Check sheet for the modelled part. Datum: model origin and axes. Units: mm. A direction names the side the tool comes from. Round coordinates to 2 decimals unless told otherwise and drop trailing zeros. Write each loop counter-clockwise with the first axis right and the second up, starting at its lowest first coordinate (ties: lowest second). Pieces come first, ordered by that corner, then holes.
Item 1: Section check C-C, the plane x = 0. Record the cut outline in (y, z).
Item 2: Section check A-A, the plane x = -9.5. Record the cut outline in (y, z).
Item 3: Section check D-D, the plane y = -1. Record the cut outline in (x, z).
Item 4: Depth check by flat-ended pin: pin 1 (0.6 mm diameter, centred on x = -14.5, z = 25, fed in from -Y); pin 2 (1 mm diameter, centred on x = -8, z = 12, fed in from -Y); pin 3 (1 mm diameter, centred on x = -14, z = 23, fed in from +Y). Enter the tip coordinate at first touch or a pass-through.
Item 5: Material ranges on line 1 along X through (y, z) = (26, 47.5); line 2 along Y through (x, z) = (0, 39); line 3 along Y through (x, z) = (10, 34.5), recorded low to high.
Item 6: Set-up check for faces 4 (the flat face through (-15, -28.721, 26)), 5 (the flat face through (29, -7, 0)), 6 (the flat face through (29, -7, 51.669)), 7 (the flat face through (-16, -22.5, 26)), 8 (the flat face through (-15.334, 24, 26)): record each of +Z, -Z, +X, -X, +Y, -Y from which the full face is reachable in a straight line by a thin tool's end or side.
Item 7: Release check for a two-part mould opening along X. For faces 1 (the flat face through (-14, 26.5, 26)), 2 (the flat face through (-15, 28.721, 26)), 3 (the flat face through (-17.334, 26, 26)) record: pulls with the +X half, pulls with the -X half, needs draft (parallel to the pull), parting line crosses it, or undercut.
Item 8: Section check B-B, the plane z = 31. Record the cut outline in (x, y).
from build123d import *

# Parameters (mm, degrees)
F1_DEPTH = 51.669
F3_DEPTH = 51.669


with BuildPart() as f1:
    # F0 (on Top) → F1 (new body)
    with BuildSketch(Plane.XY):
        with BuildLine():
            ThreePointArc((-13.334302, 26.5), (29.665698, 0), (-13.334302, -26.5))
            Line((-13.334302, -26.5), (-13.334302, -28.721077))
            ThreePointArc((-13.334302, -28.721077), (31.6655, 0), (-13.334302, 28.721077))
            Line((-13.334302, 28.721077), (-13.334302, 26.5))
        make_face()
    extrude(amount=F1_DEPTH)

    # F2 (on face) → F3 (join)
    with BuildSketch(Plane.XY.offset(51.669)):
        Polygon((-15.334302, 26.5), (-13.334302, 26.5), (-13.334302, 28.721077), (-17.334302, 28.721077), (-17.334302, 26.5), (-17.334302, 22.5), (-15.334302, 22.5), align=None)
        with BuildLine():
            Line((-11.334302, 22.5), (-11.334302, 27.415091))
            ThreePointArc((-11.334302, 27.415091), (-12.342786, 26.976087), (-13.334302, 26.5))
            Line((-13.334302, 26.5), (-13.334302, 22.5))
            Line((-13.334302, 22.5), (-11.334302, 22.5))
        make_face()
    extrude(amount=-F3_DEPTH)

    # F4: F1 across plane


with BuildPart() as f1_1:
    add(f1.part)
    add(f1.part.mirror(Plane.XZ))


solid = f1_1.part
Values found:
1. outline: (-31.67, 0) - (-29.67, 0) - (-29.67, 51.67) - (-31.67, 51.67) - close; (29.67, 0) - (31.67, 0) - (31.67, 51.67) - (29.67, 51.67) - close
2. outline: (-30.21, 0) - (-28.1, 0) - (-28.1, 51.67) - (-30.21, 51.67) - close; (28.1, 0) - (30.21, 0) - (30.21, 51.67) - (28.1, 51.67) - close
3. outline: (29.65, 0) - (31.65, 0) - (31.65, 51.67) - (29.65, 51.67) - close
4. pin 1: stops at y = -28.72
4. pin 2: stops at y = -30.76
4. pin 3: stops at y = 28.72
5. line 1: x = -17.33 to -15.33, -13.33 to -11.33, 14.28 to 18.07
5. line 2: y = -31.67 to -29.67, 29.67 to 31.67
5. line 3: y = -30.05 to -27.93, 27.93 to 30.05
6. face 4: +Z, -Z, -X, -Y
6. face 5: -Z, +X, -X, +Y, -Y
6. face 6: +Z, +X, -X, +Y, -Y
6. face 7: +Z, -Z, -X
6. face 8: +Z, -Z
7. face 1: undercut
7. face 2: needs draft
7. face 3: pulls with the -X half
8. outline: (-17.33, -28.72) - (-13.33, -28.72) arc R31.67 ccw (long way) to (-13.33, 28.72) - (-17.33, 28.72) - (-17.33, 22.5) - (-15.33, 22.5) - (-15.33, 26.5) - (-13.33, 26.5) - (-13.33, 22.5) - (-11.33, 22.5) - (-11.33, 27.42) arc R29.67 cw (long way) to (-11.33, -27.42) - (-11.33, -22.5) - (-13.33, -22.5) - (-13.33, -26.5) - (-15.33, -26.5) - (-15.33, -22.5) - (-17.33, -22.5) - close
